The listing builds one solid part. Answer for the finished solid, in the listing's coordinates (mm). Round coordinates to 2 decimals unless told otherwise and drop trailing zeros. Answer in a Markdown table with one row per item. Add a question column.
```python
from build123d import *

# Parameters (mm, degrees)
F0_W     = 49.8404
F0_H     = 183.4444
F0_R     = 1.7272
F1_DEPTH = 2
F2_R     = 5.55625
F2_R_2   = 3.96875
F2_R_3   = 1.4732
F2_R_4   = 1.016
F3_DEPTH = 25


with BuildPart() as f1:
    # F0 (on Top) → F1 (new body)
    with BuildSketch(Plane.XY):
        with Locations((21.9202, 88.7222)):
            Rectangle(F0_W, F0_H)
        with Locations((5.8754, 13.5123)):
            Circle(F0_R, mode=Mode.SUBTRACT)
        with Locations((5.8754, 30.2256)):
            Circle(F0_R, mode=Mode.SUBTRACT)
        with Locations((18.542, 8.1355)):
            Circle(F0_R, mode=Mode.SUBTRACT)
        with Locations((18.542, 18.8891)):
            Circle(F0_R, mode=Mode.SUBTRACT)
        with Locations((18.542, 24.8488)):
            Circle(F0_R, mode=Mode.SUBTRACT)
        with Locations((18.542, 35.6024)):
            Circle(F0_R, mode=Mode.SUBTRACT)
        with Locations((18.542, 41.5621)):
            Circle(F0_R, mode=Mode.SUBTRACT)
        with Locations((5.8754, 46.9389)):
            Circle(F0_R, mode=Mode.SUBTRACT)
        with Locations((5.8754, 63.6522)):
            Circle(F0_R, mode=Mode.SUBTRACT)
        with Locations((5.8754, 80.3655)):
            Circle(F0_R, mode=Mode.SUBTRACT)
        with Locations((18.542, 52.3157)):
            Circle(F0_R, mode=Mode.SUBTRACT)
        with Locations((18.542, 58.2754)):
            Circle(F0_R, mode=Mode.SUBTRACT)
        with Locations((18.542, 69.029)):
            Circle(F0_R, mode=Mode.SUBTRACT)
        with Locations((18.542, 74.9887)):
            Circle(F0_R, mode=Mode.SUBTRACT)
        with Locations((18.542, 85.7423)):
            Circle(F0_R, mode=Mode.SUBTRACT)
        with Locations((22.6394, 13.5123)):
            Circle(F0_R, mode=Mode.SUBTRACT)
        with Locations((22.6394, 30.2256)):
            Circle(F0_R, mode=Mode.SUBTRACT)
        with Locations((35.306, 8.1355)):
            Circle(F0_R, mode=Mode.SUBTRACT)
        with Locations((35.306, 18.8891)):
            Circle(F0_R, mode=Mode.SUBTRACT)
        with Locations((35.306, 24.8488)):
            Circle(F0_R, mode=Mode.SUBTRACT)
        with Locations((35.306, 35.6024)):
            Circle(F0_R, mode=Mode.SUBTRACT)
        with Locations((35.306, 41.5621)):
            Circle(F0_R, mode=Mode.SUBTRACT)
        with Locations((22.6394, 46.9389)):
            Circle(F0_R, mode=Mode.SUBTRACT)
        with Locations((22.6394, 63.6522)):
            Circle(F0_R, mode=Mode.SUBTRACT)
        with Locations((22.6394, 80.3655)):
            Circle(F0_R, mode=Mode.SUBTRACT)
        with Locations((35.306, 52.3157)):
            Circle(F0_R, mode=Mode.SUBTRACT)
        with Locations((35.306, 58.2754)):
            Circle(F0_R, mode=Mode.SUBTRACT)
        with Locations((35.306, 69.029)):
            Circle(F0_R, mode=Mode.SUBTRACT)
        with Locations((35.306, 74.9887)):
            Circle(F0_R, mode=Mode.SUBTRACT)
        with Locations((35.306, 85.7423)):
            Circle(F0_R, mode=Mode.SUBTRACT)
        with Locations((5.8754, 97.0788)):
            Circle(F0_R, mode=Mode.SUBTRACT)
        with Locations((5.8754, 113.7921)):
            Circle(F0_R, mode=Mode.SUBTRACT)
        with Locations((5.8754, 130.5054)):
            Circle(F0_R, mode=Mode.SUBTRACT)
        with Locations((18.542, 91.702)):
            Circle(F0_R, mode=Mode.SUBTRACT)
        with Locations((18.542, 102.4556)):
            Circle(F0_R, mode=Mode.SUBTRACT)
        with Locations((18.542, 108.4153)):
            Circle(F0_R, mode=Mode.SUBTRACT)
        with Locations((18.542, 119.1689)):
            Circle(F0_R, mode=Mode.SUBTRACT)
        with Locations((18.542, 125.1286)):
            Circle(F0_R, mode=Mode.SUBTRACT)
        with Locations((5.8754, 147.2187)):
            Circle(F0_R, mode=Mode.SUBTRACT)
        with Locations((5.8754, 163.932)):
            Circle(F0_R, mode=Mode.SUBTRACT)
        with Locations((18.542, 135.8822)):
            Circle(F0_R, mode=Mode.SUBTRACT)
        with Locations((18.542, 141.8419)):
            Circle(F0_R, mode=Mode.SUBTRACT)
        with Locations((18.542, 152.5955)):
            Circle(F0_R, mode=Mode.SUBTRACT)
        with Locations((18.542, 158.5552)):
            Circle(F0_R, mode=Mode.SUBTRACT)
        with Locations((18.542, 169.3088)):
            Circle(F0_R, mode=Mode.SUBTRACT)
        with Locations((22.6394, 97.0788)):
            Circle(F0_R, mode=Mode.SUBTRACT)
        with Locations((22.6394, 113.7921)):
            Circle(F0_R, mode=Mode.SUBTRACT)
        with Locations((22.6394, 130.5054)):
            Circle(F0_R, mode=Mode.SUBTRACT)
        with Locations((35.306, 91.702)):
            Circle(F0_R, mode=Mode.SUBTRACT)
        with Locations((35.306, 102.4556)):
            Circle(F0_R, mode=Mode.SUBTRACT)
        with Locations((35.306, 108.4153)):
            Circle(F0_R, mode=Mode.SUBTRACT)
        with Locations((35.306, 119.1689)):
            Circle(F0_R, mode=Mode.SUBTRACT)
        with Locations((35.306, 125.1286)):
            Circle(F0_R, mode=Mode.SUBTRACT)
        with Locations((22.6394, 147.2187)):
            Circle(F0_R, mode=Mode.SUBTRACT)
        with Locations((22.6394, 163.932)):
            Circle(F0_R, mode=Mode.SUBTRACT)
        with Locations((35.306, 135.8822)):
            Circle(F0_R, mode=Mode.SUBTRACT)
        with Locations((35.306, 141.8419)):
            Circle(F0_R, mode=Mode.SUBTRACT)
        with Locations((35.306, 152.5955)):
            Circle(F0_R, mode=Mode.SUBTRACT)
        with Locations((35.306, 158.5552)):
            Circle(F0_R, mode=Mode.SUBTRACT)
        with Locations((35.306, 169.3088)):
            Circle(F0_R, mode=Mode.SUBTRACT)
    extrude(amount=F1_DEPTH)

    # F2 (on face) → F3 (cut)
    with BuildSketch(Plane.XY.offset(2)):
        with Locations((10.5, 21.86895)):
            Circle(F2_R)
        with Locations((40.764, 113.7921)):
            Circle(F2_R_2)
        with Locations((10.5, 138.86205)):
            Circle(F2_R)
        with Locations((27.264, 155.57535)):
            Circle(F2_R)
        with Locations((40.764, 97.0788)):
            Circle(F2_R_2)
        with Locations((27.264, 122.14875)):
            Circle(F2_R)
        with Locations((27.264, 38.58225)):
            Circle(F2_R)
        with Locations((10.5, 155.57535)):
            Circle(F2_R)
        with Locations((40.764, 147.2187)):
            Circle(F2_R_2)
        with Locations((10.5, 105.43545)):
            Circle(F2_R)
        with Locations((27.264, 105.43545)):
            Circle(F2_R)
        with Locations((10.5, 88.72215)):
            Circle(F2_R)
        with Locations((27.264, 88.72215)):
            Circle(F2_R)
        with Locations((10.5, 122.14875)):
            Circle(F2_R)
        with Locations((40.764, 130.5054)):
            Circle(F2_R_2)
        with Locations((27.264, 172.28865)):
            Circle(F2_R)
        with Locations((10.5, 5.15565)):
            Circle(F2_R)
        with Locations((27.264, 5.15565)):
            Circle(F2_R)
        with Locations((27.264, 21.86895)):
            Circle(F2_R)
        with Locations((40.764, 13.5123)):
            Circle(F2_R_2)
        with Locations((27.264, 55.29555)):
            Circle(F2_R)
        with Locations((40.764, 46.9389)):
            Circle(F2_R_2)
        with Locations((10.5, 38.58225)):
            Circle(F2_R)
        with Locations((40.764, 30.2256)):
            Circle(F2_R_2)
        with Locations((40.764, 63.6522)):
            Circle(F2_R_2)
        with Locations((10.5, 172.28865)):
            Circle(F2_R)
        with Locations((27.264, 72.00885)):
            Circle(F2_R)
        with Locations((10.5, 55.29555)):
            Circle(F2_R)
        with Locations((40.764, 80.3655)):
            Circle(F2_R_2)
        with Locations((27.264, 138.86205)):
            Circle(F2_R)
        with Locations((10.5, 72.00885)):
            Circle(F2_R)
        with Locations((40.764, 163.932)):
            Circle(F2_R_2)
        with Locations((43.8404, 0)):
            Circle(F2_R_3)
        with Locations((0, 177.4444)):
            Circle(F2_R_3)
        with Locations((15, 13.5123)):
            Circle(F2_R_4)
        with Locations((33.5, 30.2256)):
            Circle(F2_R_4)
        with Locations((15, 46.9389)):
            Circle(F2_R_4)
        with Locations((33.5, 63.6522)):
            Circle(F2_R_4)
        with Locations((15, 80.3655)):
            Circle(F2_R_4)
        with Locations((33.5, 97.0788)):
            Circle(F2_R_4)
        with Locations((15, 113.7921)):
            Circle(F2_R_4)
        with Locations((33.5, 130.5054)):
            Circle(F2_R_4)
        with Locations((33.5, 163.932)):
            Circle(F2_R_4)
        with Locations((15, 147.2187)):
            Circle(F2_R_4)
        Circle(F2_R_3)
        with Locations((43.8404, 177.4444)):
            Circle(F2_R_3)
    extrude(amount=-F3_DEPTH, mode=Mode.SUBTRACT)


solid = f1.part
```
Item 1: The part is cut by section A-A, the plane x = 10.5. State how many separate pieces and enclosed holes the cut face has, and give its area (3 significant figures).
Item 2: Find the intervals of material crossed by probe 1 along X at (y, z) = (172, 0.65); probe 2 along X at (y, z) = (79, 0.4); probe 3 along X at (y, z) = (101.5, 0.2), in increasing order. Write a range as [from, to].
Item 3: A flat-ended cylindrical pin translates along its axis: P1, Ø10, axis at x = 27.26, y = 122.15, coming from the -Z side. Find the tip coordinate at first contact, or state that the pin passes through.
Resolved:
| question | item | result |
|---|---|---|
| 1 | separate pieces | 12 |
| 1 | enclosed holes | 0 |
| 1 | area | 122 mm2 |
| 2 | probe 1 | [-3, 4.95], [16.05, 21.72], [32.81, 46.84] |
| 2 | probe 2 | [-3, 4.82], [6.93, 21.58], [23.7, 37.04], [44.49, 46.84] |
| 2 | probe 3 | [-3, 6.58], [14.42, 17.1], [19.98, 23.34], [31.19, 33.87], [36.74, 46.84] |
| 3 | P1 | through |
